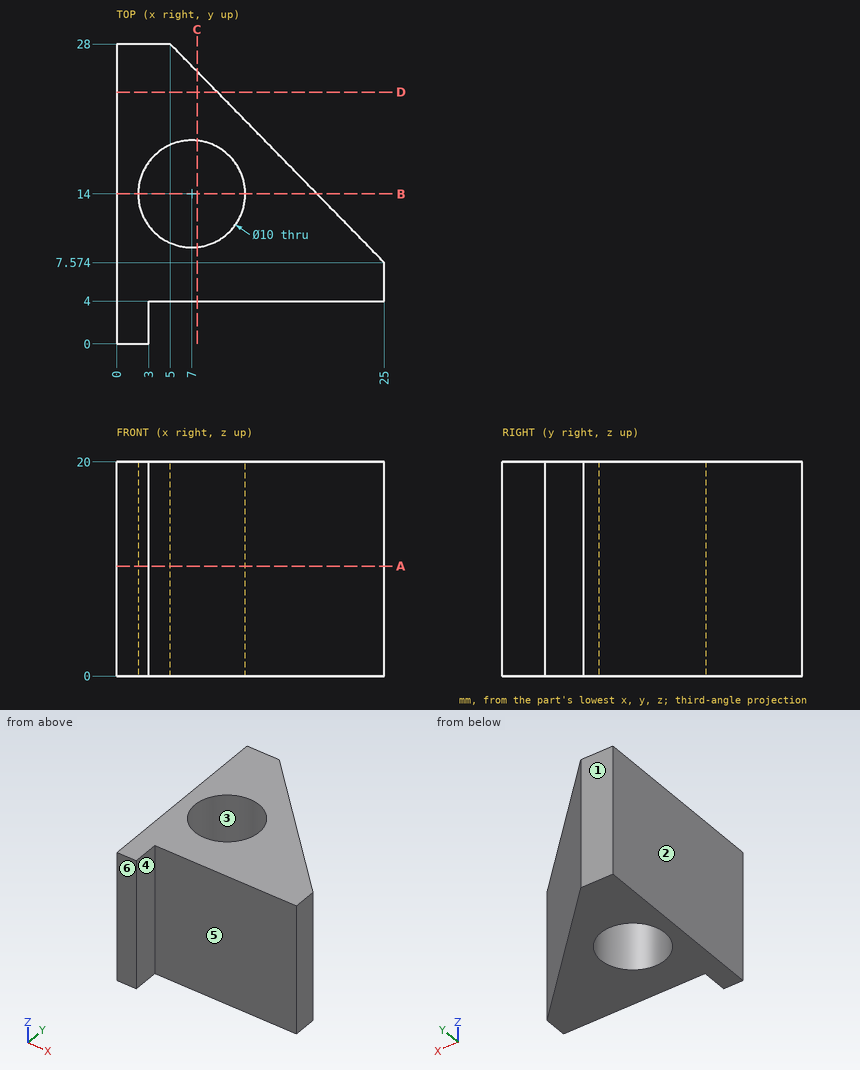
Verification items for this drawing (mm, ordinates from the low corner). A direction names the side the tool comes from. Round coordinates to 2 decimals unless told otherwise and drop trailing zeros. Loops run counter-clockwise (first coordinate to the right, second up) from the corner with the lowest first, then second, coordinate; pieces in that order, holes last. Notation, with made-up numbers: M 59,79 L 106,79 A12 cw 106,96 Z; hole C 62.25,0 d7. An arc over 180 degrees is marked long. Answer as a JSON object with one key per item and string values.
1. Scan lines: line 1 (X direction, y = 15.5, z = 17); line 2 (Y direction, x = 7, z = 5) (1 decimal); line 3 (Y direction, x = 4.5, z = 3). Record each from-to range of solid material in increasing order.
Reply:
{"line 1": "x = 0 to 2.23, 11.77 to 17.24", "line 2": "y = 4 to 9, 19 to 26", "line 3": "y = 4 to 9.67, 18.33 to 28"}
2. Section check C-C (x = 7.5). Record the boundary of the cut face in (y, z) (1 decimal), plus the area to 3 significant figures.
Reply:
{"outline": "M 4,0 L 9,0 L 9,20 L 4,20 Z; M 19,0 L 25.4,0 L 25.4,20 L 19,20 Z", "area": "230 mm²"}
3. Gauge pin test, flat ends, axial feed: P1, Ø1, axis at x = 6, z = 16, coming from the +Y side; P2, Ø1.5, axis at x = 4, z = 7.5, coming from the -Y side; P3, Ø4.5, axis at y = 1.5, z = 6.5, coming from the +X side. Record the tip position at first contact, or that the pin passes through.
Reply:
{"P1": "stops at y = 27.49", "P2": "stops at y = 4", "P3": "stops at x = 3"}
4. Section check A-A (z = 10.25). Record the boundary of the cut face in (x, y) (1 decimal).
Reply:
{"outline": "M 0,0 L 3,0 L 3,4 L 25,4 L 25,7.6 L 5,28 L 0,28 Z; hole C 7,14 d10"}
5. Mould release check, pull along X, two halves, no side actions. Record for the marked faces 1, 2, 3 and 4: pulls with the +X half, pulls with the -X half, needs draft (parallel to the pull), parting line crosses it, or undercut.
Reply:
{"face 1": "needs draft", "face 2": "pulls with the -X half", "face 3": "undercut", "face 4": "pulls with the +X half"}
6. Access from +Z, -Z, +X, -X, +Y, -Y to the whole of each face (thin tool, end or side, straight path). Record for the marked faces 5 and 6.
Reply:
{"face 5": "+Z, -Z, +X, -Y", "face 6": "+Z, -Z, +X, -X, -Y"}
7. Section check D-D (y = 23.5). Record the boundary of the cut face in (x, z), plus the area to 3 significant figures.
Reply:
{"outline": "M 0,0 L 9.41,0 L 9.41,20 L 0,20 Z", "area": "188 mm²"}
8. Section check B-B (y = 14). Record the boundary of the cut face in (x, z).
Reply:
{"outline": "M 0,0 L 2,0 L 2,20 L 0,20 Z; M 12,0 L 18.71,0 L 18.71,20 L 12,20 Z"}
